Geometry check sheet. Reference: the model listing, model coordinates, mm. Face numbers are marked on the shaded views. A direction names the side the tool comes from. Give positions to 0.01 mm unless a question says otherwise; leave off trailing zeros. Order: outer loops, then holes, each group sorted by start corner. A loop starts at its lowest first (then second) coordinate and runs counter-clockwise, first axis right, second up.
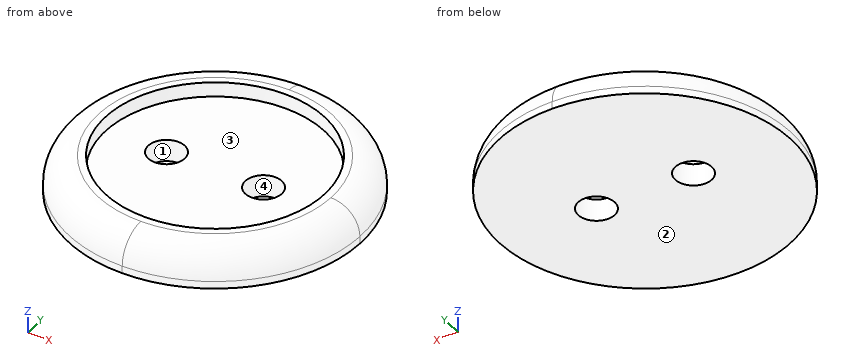
from build123d import *

# Parameters (mm, degrees)
F1_DEPTH = 2.5
F0_R     = 1.25
F2_DEPTH = 1.5
F3_R     = 2


with BuildPart() as f1:
    # F0 (on Top) → F1 (new body)
    with BuildSketch(Plane.XY):
        with BuildLine():
            ThreePointArc((0, 7.5), (5.3033008589, 5.3033008589), (7.5, 0))
            ThreePointArc((7.5, 0), (5.3033008589, -5.3033008589), (0, -7.5))
            Line((0, -7.5), (0, -10))
            ThreePointArc((0, -10), (7.0710678119, -7.0710678119), (10, 0))
            ThreePointArc((10, 0), (7.0710678119, 7.0710678119), (0, 10))
            Line((0, 10), (0, 7.5))
        make_face()
        with BuildLine():
            ThreePointArc((0, -7.5), (-7.5, 0), (0, 7.5))
            Line((0, 7.5), (0, 10))
            ThreePointArc((0, 10), (-10, 0), (0, -10))
            Line((0, -10), (0, -7.5))
        make_face()
    extrude(amount=F1_DEPTH)

    # F0 (on Top) → F2 (join)
    with BuildSketch(Plane.XY):
        with BuildLine():
            Line((0, -7.5), (0, 7.5))
            ThreePointArc((0, 7.5), (-7.5, 0), (0, -7.5))
        make_face()
        with Locations((-3.3498867415, 0)):
            Circle(F0_R, mode=Mode.SUBTRACT)
        with BuildLine():
            ThreePointArc((0, -7.5), (5.3033008589, -5.3033008589), (7.5, 0))
            ThreePointArc((7.5, 0), (5.3033008589, 5.3033008589), (0, 7.5))
            Line((0, 7.5), (0, -7.5))
        make_face()
        with Locations((3.3498867415, 0)):
            Circle(F0_R, mode=Mode.SUBTRACT)
    extrude(amount=F2_DEPTH)

    # F3
    f3_edges = [f1.edges().sort_by_distance(p)[0] for p in [
        (-10, 0, 2.5),
    ]]
    fillet(f3_edges, radius=F3_R)


solid = f1.part
Item 1: Gauge pin test, flat end, axial feed: pin 1 (7.5 mm diameter, centred on x = -3, y = 0.5, fed in from +Z). Record the tip position at first contact, or that the pin passes through.
Reported:
pin 1: stops at z = 1.5
Item 2: Sectioned sample at A-A (z = 1.2). Enter the section's corners in (x, y).
Reported:
outline: circle Ø19.75 at (0, 0); hole circle Ø2.5 at (-3.35, 0); hole circle Ø2.5 at (3.35, 0)
Item 3: Draft check along Y on the marked faces 1 and 2. Enter one of: released by +Y, released by -Y, zero draft, split by the parting line, or undercut.
Reported:
face 1: undercut
face 2: zero draft
Item 4: Scan lines: L1, parallel to X at y = 1, z = 1; L2, parallel to Z at x = -6.25, y = -1; L3, parallel to X at y = 6, z = 1.85. Record each from-to range of solid material in increasing order.
Reported:
L1: x = -9.89 to -4.1, -2.6 to 2.6, 4.1 to 9.89
L2: z = 0 to 1.5
L3: x = -7.33 to -4.5, 4.5 to 7.33
Item 5: Set-up check for the marked faces 3 and 4: record each of +Z, -Z, +X, -X, +Y, -Y from which the full face is reachable in a straight line by a thin tool's end or side.
Reported:
face 3: +Z
face 4: +Z, -Z
